The model under review builds one solid part; all positions refer to its coordinate system, in mm. Face numbers are marked on the shaded views. A direction names the side the tool comes from. Round coordinates to 2 decimals unless told otherwise and drop trailing zeros. Write each loop counter-clockwise with the first axis right and the second up, starting at its lowest first coordinate (ties: lowest second). Pieces come first, ordered by that corner, then holes. Notation, with made-up numbers: (27.5, -16) -> (70.5, -16) arc R22 cw to (70.5, -8) -> close; hole circle Ø2 at (17, -35.5). An arc over 180 degrees is marked (long way). Return JSON: item names as keys, results as strings. Group by question number.
1. Take a section at B-B, the plane y = -82. Write out the cut boundary in (x, z).
2. Take a section at D-D, the plane z = 73. Write out the cut boundary in (x, y).
3. Take a section at C-C, the plane x = 22.5. Write out the cut boundary in (y, z), then the cut area to 3 significant figures.
4. Take a section at A-A, the plane x = -5. Write out the cut boundary in (y, z).
5. Mouldability with a two-part tool opening along Y and no side actions: class the marked faces 4, 5 and 6 as pulls with the +Y half, pulls with the -Y half, needs draft (parallel to the pull), parting line crosses it, or undercut.
6. For line 1 along Z through (x, y) = (53, -73.5); line 2 along Y through (x, z) = (8.5, 32); line 3 along Y through (x, z) = (86, 65.5), list the stretches that pass through material, from the lowest coordinate up. Write a range as from..to.
7. Tool access review of the marked faces 1, 2 and 3: name each direction out of +Z, -Z, +X, -X, +Y, -Y from which nothing blocks a thin tool from reaching the whole face with its end or side.
8. Clearance check with flat-ended pins moving along their axes: P1, Ø2, axis at x = 14, z = 45.5, coming from the -Y side; P2, Ø6, axis at x = -14, z = -32, coming from the +Y side; P3, Ø6, axis at x = 34.5, y = -76.5, coming from the -Z side. State where each tip first meets the part, or that it passes through.
from build123d import *

# Parameters (mm, degrees)
F0_W     = 100
F0_H     = 100
F1_DEPTH = 100
F2_R     = 35
F3_DEPTH = 70
F4_R     = 35
F5_DEPTH = 70


with BuildPart() as f1:
    # F0 (on Front) → F1 (new body)
    with BuildSketch(Plane.XZ):
        with Locations((50, 50)):
            Rectangle(F0_W, F0_H)
    extrude(amount=F1_DEPTH)

    # F2 (on face) → F3 (join)
    with BuildSketch(Plane(origin=(0, 0, 0), x_dir=(1, 0, 0), z_dir=(0, 0, -1))):
        Circle(F2_R)
    extrude(amount=F3_DEPTH)

    # F4 (on face) → F5 (join)
    with BuildSketch(Plane.XZ.offset(100)):
        Circle(F4_R)
    extrude(amount=F5_DEPTH)


solid = f1.part
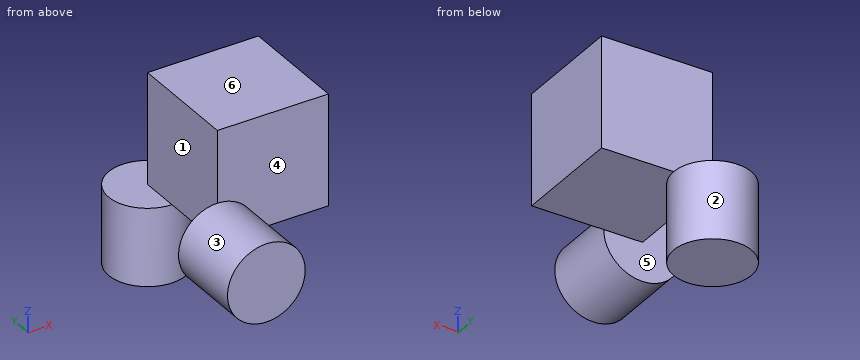
Output:
{
 "1": {"outline": "(0, 0) -> (100, 0) -> (100, 100) -> (0, 100) -> close"},
 "2": {"outline": "(0, -100) -> (100, -100) -> (100, 0) -> (0, 0) -> close"},
 "3": {"outline": "(-170, -26.81) -> (-100, -26.81) -> (-100, 0) -> (-26.81, 0) -> (-26.81, -70) -> (26.81, -70) -> (26.81, 0) -> (0, 0) -> (0, 100) -> (-100, 100) -> (-100, 26.81) -> (-170, 26.81) -> close", "area": "17,500 mm^2"},
 "4": {"outline": "(-170, -34.64) -> (-100, -34.64) -> (-100, 34.64) -> (-170, 34.64) -> close; (-34.64, -70) -> (34.64, -70) -> (34.64, 0) -> (-34.64, 0) -> close"},
 "5": {"face 4": "pulls with the -Y half", "face 5": "undercut", "face 6": "needs draft"},
 "6": {"line 1": "z = 0..100", "line 2": "y = -170..0", "line 3": "y = -100..0"},
 "7": {"face 1": "+Z, -X, +Y", "face 2": "-Z", "face 3": "-Y"},
 "8": {"P1": "stops at y = -100", "P2": "stops at y = 33.23", "P3": "stops at z = 0"}
}
